```python
from build123d import *

# Parameters (mm, degrees)
SKETCH1_W           = 22
SKETCH1_H           = 120
BOSS_EXTRUDE1_DEPTH = 39
SKETCH2_OUTSIDE_W   = 49.616
SKETCH2_OUTSIDE_H   = 147.616
CUT_EXTRUDE1_DEPTH  = 73.40165744
FILLET1_R           = 5
CUT_EXTRUDE2_DEPTH  = 73.40165744
SKETCH4_W           = 96.947441117
SKETCH4_H           = 39
BOSS_EXTRUDE2_DEPTH = 5
SKETCH5_W           = 4
SKETCH5_H           = 96.947441117
CUT_EXTRUDE3_DEPTH  = 74.328030111
SKETCH6_W           = 4
SKETCH6_H           = 96.947441117
CUT_EXTRUDE4_DEPTH  = 74.328030111
SKETCH7_R           = 2
CUT_EXTRUDE5_DEPTH  = 73.560319735
SKETCH8_W           = 5
SKETCH8_H           = 26
CUT_EXTRUDE6_DEPTH  = 73.560319735


with BuildPart() as part:
    # Sketch1 → Boss-Extrude1 (new body)
    with BuildSketch(Plane(origin=(0, 0, 0), x_dir=(1, 0, 0), z_dir=(0, 1, 0))):
        Rectangle(SKETCH1_W, SKETCH1_H)
    extrude(amount=BOSS_EXTRUDE1_DEPTH)

    # Sketch2 outside → Cut-Extrude1 (cut, through all)
    with BuildSketch(Plane(origin=(0, 39, 0), x_dir=(1, 0, 0), z_dir=(0, 1, 0))):
        Rectangle(SKETCH2_OUTSIDE_W, SKETCH2_OUTSIDE_H)
        Polygon((0, 60), (-11, 40.947441117), (-11, -60), (11, -60), (11, 40.947441117), align=None, mode=Mode.SUBTRACT)
    extrude(amount=-CUT_EXTRUDE1_DEPTH, mode=Mode.SUBTRACT)

    # Fillet1
    fillet1_edges = [part.edges().sort_by_distance(p)[0] for p in [
        (0, 19.5, -60),
    ]]
    fillet(fillet1_edges, radius=FILLET1_R)

    # Sketch3 → Cut-Extrude2 (cut, through all)
    with BuildSketch(Plane(origin=(0, 39, 0), x_dir=(1, 0, 0), z_dir=(0, 1, 0))):
        Polygon((-11, 36.947441117), (-7, 36.947441117), (-7, 47.875644347), (-11, 40.947441117), align=None)
        Polygon((7, 47.875644347), (11, 40.947441117), (11, 36.947441117), (7, 36.947441117), align=None)
    extrude(amount=-CUT_EXTRUDE2_DEPTH, mode=Mode.SUBTRACT)

    # Sketch4 → Boss-Extrude2 (add)
    with BuildSketch(Plane(origin=(11, 0, 0), x_dir=(0, 0, -1), z_dir=(1, 0, 0))):
        with Locations((-11.526279442, 19.5)):
            Rectangle(SKETCH4_W, SKETCH4_H)
    extrude(amount=BOSS_EXTRUDE2_DEPTH)

    # Sketch5 → Cut-Extrude3 (cut, through all)
    with BuildSketch(Plane(origin=(0, 39, 0), x_dir=(1, 0, 0), z_dir=(0, 1, 0))):
        with Locations((-9, -11.526279442)):
            Rectangle(SKETCH5_W, SKETCH5_H)
    extrude(amount=-CUT_EXTRUDE3_DEPTH, mode=Mode.SUBTRACT)

    # Sketch6 → Cut-Extrude4 (cut, through all)
    with BuildSketch(Plane(origin=(0, 39, 0), x_dir=(1, 0, 0), z_dir=(0, 1, 0))):
        with Locations((14, -11.526279442)):
            Rectangle(SKETCH6_W, SKETCH6_H)
    extrude(amount=-CUT_EXTRUDE4_DEPTH, mode=Mode.SUBTRACT)

    # Sketch7 → Cut-Extrude5 (cut, through all)
    with BuildSketch(Plane(origin=(0, 39, 0), x_dir=(1, 0, 0), z_dir=(0, 1, 0))):
        with Locations(Location((0, 46, 0), (0, 0, 270))):
            Circle(SKETCH7_R)
    extrude(amount=-CUT_EXTRUDE5_DEPTH, mode=Mode.SUBTRACT)

    # Sketch8 → Cut-Extrude6 (cut, through all)
    with BuildSketch(Plane(origin=(0, 39, 0), x_dir=(1, 0, 0), z_dir=(0, 1, 0))):
        with Locations((9.5, 23.947441117)):
            Rectangle(SKETCH8_W, SKETCH8_H)
    extrude(amount=-CUT_EXTRUDE6_DEPTH, mode=Mode.SUBTRACT)


solid = part.part
```
Model file for the job. Use its own axes, mm. A direction names the side the tool comes from. Give positions to 0.01 mm unless a question says otherwise; leave off trailing zeros. Loops run counter-clockwise (first coordinate to the right, second up) from the corner with the lowest first, then second, coordinate; pieces in that order, holes last. Notation, with made-up numbers: (44.5, -29.75) -> (86.5, -29.75) arc R25 cw to (86.5, -1.75) -> close; hole circle Ø2 at (82, 27.5). An arc over 180 degrees is marked (long way). Use CSV: the item, a comma, the result in double quotes. Start each with the question number.
1) Tool access for faces 4 (the flat face through (2, 19, 60)), 5 (the flat face through (9, 20, -10.947)): list every direction of +Z, -Z, +X, -X, +Y, -Y with a clear straight run to the whole face (end or side of a thin tool).
2) Mould opens along Z. For faces 1 (the flat face through (7, 20, -29)), 2 (the cylindrical face through (0, 20, -48)), 3 (the flat face through (5.68, 19.77, -50.16)) say: released by +Z, released by -Z, zero draft, split by the parting line, or undercut.
3) Slice it at C-C on y = 36.5. Give the cut face in (x, z).
4) Wall check: line 1 (X direction, y = 27, z = -46); line 2 (X direction, y = 14, z = -13); line 3 (Z direction, x = 0.75, y = 9.5). Give the ranges that are in metal, low to high.
5) Flat gauge pins, fed straight in: pin 1 Ø2 at (x, y) = (5, 12.5) entering from -Z; pin 2 Ø5 at (x, y) = (4, 10) entering from -Z; pin 3 Ø2.5 at (x, y) = (9, 14) entering from -Z. Where does each tip first touch, or does it go through?
6) Slice it at B-B on z = -46. Give the cut face in (x, y), plus the area to 3 significant figures.
7) Slice it at A-A on x = 0. Give the cut face in (y, z).
Computed values:
1,face 4,"+Z, +X, -X, +Y, -Y"
1,face 5,"-Z, +X, +Y, -Y"
2,face 1,"zero draft"
2,face 2,"undercut"
2,face 3,"released by -Z"
3,outline,"(-7, -47.88) -> (-4.33, -52.5) arc R5 ccw to (4.33, -52.5) -> (7, -47.88) -> (7, -10.95) -> (12, -10.95) -> (12, 60) -> (-7, 60) -> close; hole circle Ø4 at (0, -46)"
4,line 1,"x = -7 to -2, 2 to 7"
4,line 2,"x = -7 to 7"
4,line 3,"z = -54.94 to -47.85, -44.15 to 60"
5,pin 1,"stops at z = -53"
5,pin 2,"stops at z = -54.77"
5,pin 3,"stops at z = -10.95"
6,outline,"(-7, 0) -> (-2, 0) -> (-2, 39) -> (-7, 39) -> close; (2, 0) -> (7, 0) -> (7, 39) -> (2, 39) -> close"
6,area,"390 mm^2"
7,outline,"(0, -55) -> (39, -55) -> (39, -48) -> (0, -48) -> close; (0, -44) -> (39, -44) -> (39, 60) -> (0, 60) -> close"
